Verification items for the finished model (mm, model axes). Give positions to 0.01 mm unless a question says otherwise; leave off trailing zeros. Loops run counter-clockwise (first coordinate to the right, second up) from the corner with the lowest first, then second, coordinate; pieces in that order, holes last. Notation, with made-up numbers: (83.5, 81) -> (124.5, 81) arc R24 ccw to (124.5, 117) -> close; hole circle Ø4 at (10, -35). An arc over 180 degrees is marked (long way). Answer in a Markdown table with one row per item. Add a question column.
Q1. Section check D-D on x = 28.5. Enter the section's corners in (y, z).
Q2. Gauge pin test, flat ends, axial feed: P1, Ø1.5, axis at x = -16, z = 1.5, coming from the -Y side; P2, Ø12, axis at x = -23.5, y = 23.5, coming from the +Z side. Record the tip position at first contact, or that the pin passes through.
Q3. Release check for a two-part mould opening along Y. For faces 1 (the face through (-6.94, 31.24, 2.46)), 2 (the face through (17.07, 0.65, 2.46)), 3 (the face through (0, 0, 0)), 4 (the face through (20.05, -19.07, 2.54)) record: pulls with the +Y half, pulls with the -Y half, needs draft (parallel to the pull), parting line crosses it, or undercut.
Q4. Material ranges on probe 1 along Y at (x, z) = (0, 3.1); probe 2 along X at (y, z) = (1, 3.95); probe 3 along Y at (x, z) = (18, 2.75), recorded low to high.
Q5. Section check B-B on y = -3.5. Enter the section's corners in (x, z).
Q6. Section check C-C on y = -24.5. Enter the section's corners in (x, z).
Q7. Section check A-A on x = 15.5. Enter the section's corners in (y, z).
Autodesk Inventor part; units mm, degrees
ref_plane "YZ Plane" through (0, 0, 0) normal (1, 0, 0) x (0, 1, 0)
ref_plane "XZ Plane" through (0, 0, 0) normal (0, 1, 0) x (-1, 0, 0)
ref_plane "XY Plane" through (0, 0, 0) normal (0, 0, 1) x (1, 0, 0)
sketch "Sketch1" plane through (0, 0, 0) normal (0, 0, 1) x (1, 0, 0)
  circle A0 centre (0, 0) radius 32
  circle A1 centre (-15.5, 0) radius 1.7
  circle A2 centre (15.5, 0) radius 1.7
  circle A3 centre (0, -9.9) radius 8
  circle A4 centre (0, 0) radius 18.5
  dimension "d10" = 16
  dimension "d13" = 64
  dimension "d14" = 37
extrude "Extrusion3" add sketch "Sketch1" along normal blind 5 contours A0 | A4
sketch "Sketch2" plane through (0, 0, 5) normal (0, 0, 1) x (1, 0, 0)
  circle A0 centre (0, -9.9) radius 8
  circle A1 centre (15.5, 0) radius 1.7
  circle A2 centre (-15.5, 0) radius 1.7
  circle A3 centre (0, 0) radius 32
  circle A4 centre (0, 24) radius 1.8
  line L0 (0, 0) -> (-22.6274, -22.6274)
  line L1 (0, 0) -> (-41.0301, 0)
  line L2 (-22.6274, -22.6274) -> (-18.3848, -18.3848)
  circle A5 centre (-18.3848, -18.3848) radius 1.8
  line L3 (0, 0) -> (0, 6.0561)
  circle A6 centre (18.3848, -18.3848) radius 1.8
  dimension "d15" = 3.6
  dimension "d16" = 45
  dimension "d17" = 6
  dimension "d18" = 3.6
  dimension "d21" = 24
extrude "Extrusion4" cut sketch "Sketch2" against normal up to next contours A5 L0 | L0 A5 | A4 | A6
properties part number "SUPORT STEEP 2"
Taken from the geometry:
| question | item | result |
|---|---|---|
| 1 | outline | (-14.55, 0) -> (14.55, 0) -> (14.55, 5) -> (-14.55, 5) -> close |
| 2 | P1 | stops at y = -28.13 |
| 2 | P2 | stops at z = 5 |
| 3 | face 1 | parting line crosses it |
| 3 | face 2 | undercut |
| 3 | face 3 | needs draft |
| 3 | face 4 | undercut |
| 4 | probe 1 | y = -32 to -17.9, -1.9 to 22.2, 25.8 to 32 |
| 4 | probe 2 | x = -31.98 to -16.87, -14.13 to 14.13, 16.87 to 31.98 |
| 4 | probe 3 | y = -26.46 to -20.14, -16.63 to 26.46 |
| 5 | outline | (-31.81, 0) -> (-4.8, 0) -> (-4.8, 5) -> (-31.81, 5) -> close; (4.8, 0) -> (31.81, 0) -> (31.81, 5) -> (4.8, 5) -> close |
| 6 | outline | (-20.59, 0) -> (20.59, 0) -> (20.59, 5) -> (-20.59, 5) -> close |
| 7 | outline | (-28, 0) -> (-1.7, 0) -> (-1.7, 5) -> (-28, 5) -> close; (1.7, 0) -> (28, 0) -> (28, 5) -> (1.7, 5) -> close |
